Autodesk Inventor part; units mm, degrees
ref_plane "YZ Plane" through (0, 0, 0) normal (1, 0, 0) x (0, 1, 0)
ref_plane "XZ Plane" through (0, 0, 0) normal (0, 1, 0) x (-1, 0, 0)
ref_plane "XY Plane" through (0, 0, 0) normal (0, 0, 1) x (1, 0, 0)
sketch "Sketch2" plane through (0, 0, 0) normal (0, 0, 1) x (1, 0, 0)
  circle A0 centre (0, 0) radius 15
  dimension "d0" = 30
extrude "Extrusion1" add sketch "Sketch2" against normal blind 5
sketch "Sketch3" plane through (0, 0, 0) normal (0, 0, 1) x (1, 0, 0)
  circle A0 centre (0, 0) radius 9
  dimension "d3" = 18
extrude "Extrusion2" add sketch "Sketch3" against normal blind 17
sketch "Sketch4" plane through (0, 0, 0) normal (0, 0, 1) x (1, 0, 0)
  circle A0 centre (0, 0) radius 5
  dimension "d6" = 10
extrude "Extrusion3" cut sketch "Sketch4" against normal blind 17
equation "\"BendRadius\" = Thickness"
equation "\"BendReliefWidth\" = Thickness"
equation "\"BendReliefDepth\" = 0.5 * Thickness"
equation "\"CornerReliefSize\" = 4 * Thickness"
equation "\"MinimumRemnant\" = 2 * Thickness"
equation "\"TransitionRadius\" = BendRadius"
equation "\"JacobiRadiusSize\" = BendRadius"
equation "\"GapSize\" = Thickness"
properties part number "Bushing_beam_stempel_long"
Geometry: final body of the model. Coordinates: model frame, mm. A direction names the side the tool comes from. Coordinates: 2 decimals unless noted, no trailing zeros. Order: outer loops, then holes, each group sorted by start corner. A loop starts at its lowest first (then second) coordinate and runs counter-clockwise, first axis right, second up. Notation, with made-up numbers: (-1.75, 18.5) -> (35.25, 18.5) arc R37 ccw to (35.25, 56.5) -> close; hole circle Ø2 at (-11, 82.5). An arc over 180 degrees is marked (long way). Write item = value, one per line.
(1) Line query: line 1 (Y direction, x = 0, z = -11.25); line 2 (Z direction, x = 11.75, y = 3.5); line 3 (X direction, y = 1, z = -11.25). Output: solid intervals per line, ascending.
Solved:
line_1 = -9 to -5, 5 to 9
line_2 = -5 to 0
line_3 = -8.94 to -4.9, 4.9 to 8.94
(2) Cut plane A-A on y = 0. Return loops of the section in (x, z), plus the area to 3 significant figures.
Solved:
outline = (-15, -5) -> (-9, -5) -> (-9, -17) -> (-5, -17) -> (-5, 0) -> (-15, 0) -> close; (5, -17) -> (9, -17) -> (9, -5) -> (15, -5) -> (15, 0) -> (5, 0) -> close
area = 196 mm²
(3) Pull-direction query (Y, two-part tool) for faces 1 (the flat face through (4, -4, -17)), 2 (the cylindrical face through (-1.172, 8.923, -10.916)), 3 (the cylindrical face through (-1.08, -4.88, -8.38)); classes: pulls with the +Y half, pulls with the -Y half, needs draft (parallel to the pull), parting line crosses it, or undercut.
Solved:
face_1 = needs draft
face_2 = parting line crosses it
face_3 = undercut
(4) Pin query (flat end, axial travel): pin 1 Ø5 at (x, z) = (-1, -13) entering from +Y; pin 2 Ø6 at (x, z) = (6.5, -12.5) entering from -Y; pin 3 Ø5 at (x, z) = (-8.5, -11.5) entering from +Y; pin 4 Ø8 at (x, y) = (0, 0) entering from -Z. Return the tip coordinate at first contact, or that it passes through.
Solved:
pin_1 = 9
pin_2 = -8.29
pin_3 = 6.71
pin_4 = through
(5) Cut plane D-D on z = -6.25. Return loops of the section in (x, y).
Solved:
outline = circle Ø18 at (0, 0); hole circle Ø10 at (0, 0)
(6) Access query for faces 4 (the flat face through (6.5, -6.5, -5)), 5 (the flat face through (-4, 4, 0)). Directions: +Z, -Z, +X, -X, +Y, -Y. A direction counts if a zero-diameter tool reaches every point of the face in a straight line with its end or side. Return the directions, or none.
Solved:
face_4 = -Z
face_5 = +Z, +X, -X, +Y, -Y
(7) Cut plane C-C on z = -4. Return loops of the section in (x, y), plus the area to 3 significant figures.
Solved:
outline = circle Ø30 at (0, 0); hole circle Ø10 at (0, 0)
area = 628 mm²
